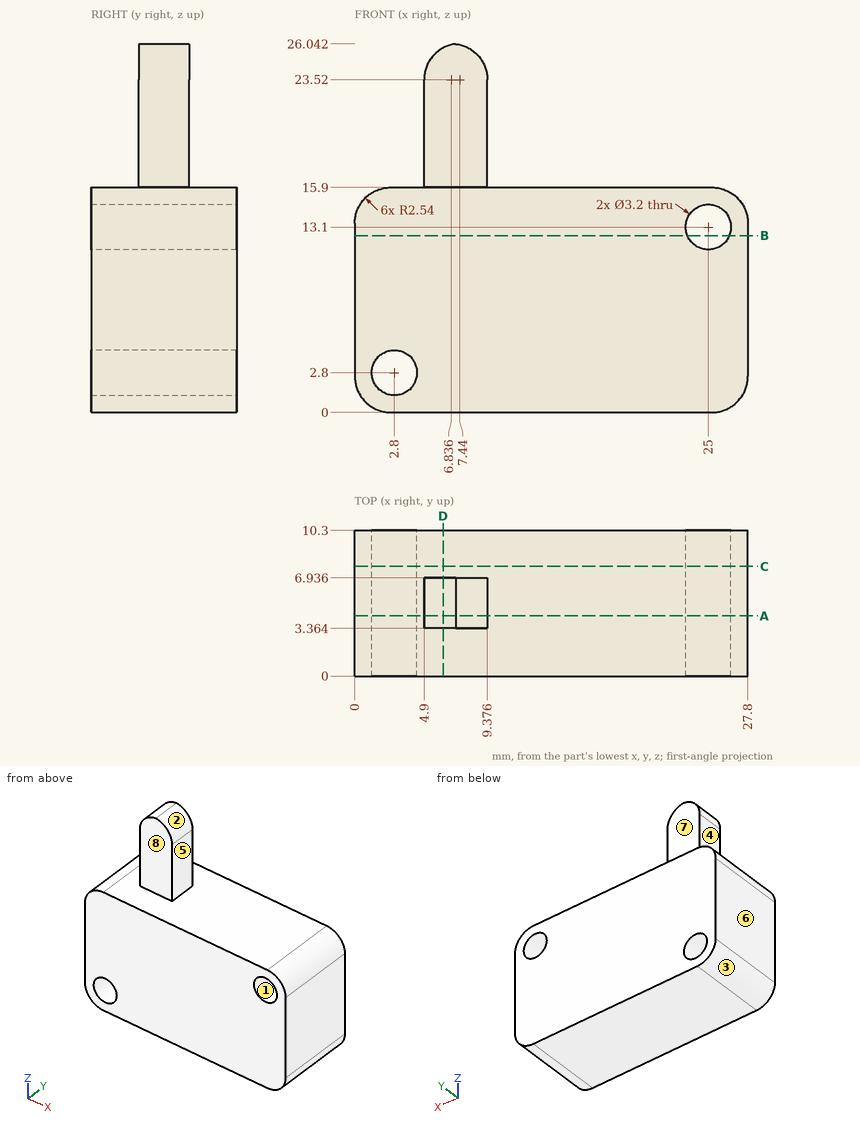
Geometry: see drawing. Coordinates: mm, zero at the bounding-box minimum. A direction names the side the tool comes from. Give positions to 0.01 mm unless a question says otherwise; leave off trailing zeros. Order: outer loops, then holes, each group sorted by start corner. A loop starts at its lowest first (then second) coordinate and runs counter-clockwise, first axis right, second up.
1. Pin query (flat end, axial travel): pin 1 Ø4 at (y, z) = (4.5, 20) entering from +X; pin 2 Ø1.1 at (y, z) = (5, 18) entering from -X; pin 3 Ø3.5 at (x, z) = (8, 22.5) entering from +Y. Return the tip coordinate at first contact, or that it passes through.
Computed:
pin 1: stops at x = 9.38
pin 2: stops at x = 4.9
pin 3: stops at y = 6.94
2. Line query: probe 1 along X at (y, z) = (6.25, 13.1); probe 2 along Z at (x, y) = (25, 5.5); probe 3 along X at (y, z) = (4.75, 2.8). Output: solid intervals per line, ascending.
Computed:
probe 1: x = 0 to 23.4, 26.6 to 27.8
probe 2: z = 0 to 11.5, 14.7 to 15.9
probe 3: x = 0 to 1.2, 4.4 to 27.8
3. Cut plane A-A (y = 4.25). Return loops of the section in (x, z), and give its area (3 significant figures).
Computed:
outline: (0, 2.54) arc R2.54 ccw to (2.54, 0) - (25.26, 0) arc R2.54 ccw to (27.8, 2.54) - (27.8, 13.36) arc R2.54 ccw to (25.26, 15.9) - (9.38, 15.9) - (9.38, 23.52) arc R2.54 ccw to (7.14, 26.04) arc R2.54 ccw to (4.9, 23.52) - (4.9, 15.9) - (2.54, 15.9) arc R2.54 ccw to (0, 13.36) - close; hole circle Ø3.2 at (2.8, 2.8); hole circle Ø3.2 at (25, 13.1)
area: 463 mm2
4. Cut plane B-B (z = 12.5). Return loops of the section in (x, y), and give its area (3 significant figures).
Computed:
outline: (0, 0) - (23.52, 0) - (23.52, 10.3) - (0, 10.3) - close; (26.48, 0) - (27.8, 0) - (27.8, 10.3) - (26.48, 10.3) - close
area: 256 mm2
5. Draft query along Z for the marked faces 1, 2 and 3. Return one class per face: released by +Z, released by -Z, zero draft, split by the parting line, or undercut.
Computed:
face 1: undercut
face 2: released by +Z
face 3: released by -Z
6. Cut plane C-C (y = 7.75). Return loops of the section in (x, z).
Computed:
outline: (0, 2.54) arc R2.54 ccw to (2.54, 0) - (25.26, 0) arc R2.54 ccw to (27.8, 2.54) - (27.8, 13.36) arc R2.54 ccw to (25.26, 15.9) - (2.54, 15.9) arc R2.54 ccw to (0, 13.36) - close; hole circle Ø3.2 at (2.8, 2.8); hole circle Ø3.2 at (25, 13.1)
7. Set-up query: the marked faces 4, 5, 6, 7 and 8. Return all of +Z, -Z, +X, -X, +Y, -Y with unobstructed straight access to the full face (end or side cutting, diameter ignored); none if empty.
Computed:
face 4: +Z, -X, +Y, -Y
face 5: +Z, +X, +Y, -Y
face 6: +Z, -Z, -X, +Y, -Y
face 7: +Z, +X, -X, +Y
face 8: +Z, +X, -X, -Y
8. Cut plane D-D (x = 6.25). Return loops of the section in (y, z) (1 decimal).
Computed:
outline: (0, 0) - (10.3, 0) - (10.3, 15.9) - (6.9, 15.9) - (6.9, 25.8) - (3.4, 25.8) - (3.4, 15.9) - (0, 15.9) - close
